Work out the finished part from the listing and answer in its coordinate system (mm). A direction names the side the tool comes from. Give positions to 0.01 mm unless a question says otherwise; leave off trailing zeros. Order: outer loops, then holes, each group sorted by start corner. A loop starts at its lowest first (then second) coordinate and runs counter-clockwise, first axis right, second up. Notation, with made-up numbers: (31.25, 34) -> (44.25, 34) arc R3 ccw to (44.25, 38) -> close; hole circle Ø11 at (49, -8). An arc over 180 degrees is marked (long way). Use a Markdown table: item, result. Add a question column.
```python
from build123d import *

# Parameters (mm, degrees)
F1_DEPTH = 63.5
F0_W     = 25.4
F0_H     = 19.05
F2_DEPTH = 25.4
F3_DEPTH = 7.9375
F5_R     = 6.35


with BuildPart() as f1:
    # F0 (on Front) → F1 (new body, symmetric)
    with BuildSketch(Plane.XZ):
        Polygon((22.225, 9.525), (-41.275, 9.525), (-41.275, -9.525), (41.275, -9.525), (41.275, 9.525), align=None)
    extrude(amount=F1_DEPTH, both=True)

    # F0 (on Front) → F2 (join, symmetric)
    with BuildSketch(Plane.XZ):
        with Locations((73.025, 52.4002)):
            Rectangle(F0_W, F0_H)
        with BuildLine():
            Line((22.225, 27.0015947561), (22.225, 9.525))
            Line((22.225, 9.525), (41.275, 9.525))
            Line((41.275, 9.525), (41.275, 27.0015947561))
            ThreePointArc((41.275, 27.0015947561), (45.8505258857, 38.1522678183), (56.9395681561, 42.8752))
            Line((56.9395681561, 42.8752), (60.325, 42.8752))
            Line((60.325, 42.8752), (60.325, 61.9252))
            Line((60.325, 61.9252), (56.837875396, 61.9252))
            add(Edge.make_bspline(
                [(56.837875396, 61.9252), (56.1791036385, 61.904913743), (55.5200497896, 61.880354768), (54.8608113135, 61.8514905975)],
                knots=[0, 0, 0, 0, 1.9281744769, 1.9281744769, 1.9281744769, 1.9281744769], degree=3))
            ThreePointArc((54.8608113135, 61.8514905975), (31.6577900146, 50.8742329652), (22.225, 27.0015947561))
        make_face()
    extrude(amount=F2_DEPTH, both=True)

    # F0 (on Front) → F3 (join, symmetric)
    with BuildSketch(Plane.XZ):
        with BuildLine():
            add(Edge.make_bspline(
                [(54.8608113135, 61.8514905975), (17.4910659658, 60.2152895251), (-20.4719474509, 44.745078984), (-41.275, 9.525)],
                knots=[1.9281744769, 1.9281744769, 1.9281744769, 1.9281744769, 111.2291206407, 111.2291206407, 111.2291206407, 111.2291206407], degree=3))
            Line((-41.275, 9.525), (22.225, 9.525))
            Line((22.225, 9.525), (22.225, 27.0015947561))
            ThreePointArc((22.225, 27.0015947561), (31.6577900146, 50.8742329652), (54.8608113135, 61.8514905975))
        make_face()
    extrude(amount=F3_DEPTH, both=True)

    # F0 (on Front) → F4 (revolve)
    with BuildSketch(Plane.XZ):
        Polygon((85.725, 66.675), (85.725, 61.9252), (85.725, 42.8752), (85.725, 38.1), (111.125, 38.1), (111.125, 66.675), align=None)
    revolve(axis=Axis((85.725, 0, 51.1358389631), (0, 0, -1)))

    # F5
    f5_edges = [f1.edges().sort_by_distance(p)[0] for p in [
        (41.275, -63.5, 0),
        (-41.275, -63.5, 0),
        (-41.275, 63.5, 0),
        (41.275, 63.5, 0),
    ]]
    fillet(f5_edges, radius=F5_R)


solid = f1.part
```
1) The part is cut by section B-B, the plane x = 84. Determine the outline of the cut face in (y, z) (3 decimals), then the cut area to 3 significant figures.
2) Flat-ended cylindrical pins translate along their axes: pin 1 (19 mm diameter, centred on y = 16, z = 15, fed in from -X) (3 decimals); pin 2 (10 mm diameter, centred on x = -17.5, y = -13.5, fed in from +Z) (3 decimals); pin 3 (18.5 mm diameter, centred on y = -6, z = 6, fed in from +X) (3 decimals); pin 4 (12 mm diameter, centred on x = 79.5, z = 53, fed in from +Y). Find the tip coordinate at first contact, or state that the pin passes through.
3) Straight lines are drawn through the part: line 1 (Y direction, x = -5.5, z = 22); line 2 (Z direction, x = -4, y = -37) (3 decimals); line 3 (X direction, y = 44, z = 0) (3 decimals). For each, find the intervals that lie inside material, in ascending order.
4) The part is cut by section A-A, the plane y = -42. Determine the outline of the cut face in (x, z) (3 decimals), then the cut area to 3 significant figures.
5) Which of the six approach directions +Z, -Z, +X, -X, +Y, -Y give full straight-line access (tool end or side, diameter ignored) to faces 1 (the flat face through (6, -7.938, 30)), 2 (the flat face through (60, 0, 42.875)), 3 (the flat face through (22.225, 17, 18))?
A:
| question | item | result |
|---|---|---|
| 1 | outline | (-25.4, 42.875) -> (-25.341, 42.875) -> (-25.341, 38.1) -> (25.341, 38.1) -> (25.341, 42.875) -> (25.4, 42.875) -> (25.4, 61.925) -> (25.341, 61.925) -> (25.341, 66.675) -> (-25.341, 66.675) -> (-25.341, 61.925) -> (-25.4, 61.925) -> close |
| 1 | area | 1,450 mm^2 |
| 2 | pin 1 | x = -41.275 |
| 2 | pin 2 | z = 9.525 |
| 2 | pin 3 | x = 41.275 |
| 2 | pin 4 | y = 25.4 |
| 3 | line 1 | -7.94 to 7.94 |
| 3 | line 2 | -9.525 to 9.525 |
| 3 | line 3 | -41.275 to 41.275 |
| 4 | outline | (-41.275, -9.525) -> (41.275, -9.525) -> (41.275, 9.525) -> (-41.275, 9.525) -> close |
| 4 | area | 1,570 mm^2 |
| 5 | face 1 | +Z, -X, -Y |
| 5 | face 2 | -Z |
| 5 | face 3 | +Z, -X, +Y |
